Verification items for the finished model (mm, model axes). Round coordinates to 2 decimals unless told otherwise and drop trailing zeros. Write each loop counter-clockwise with the first axis right and the second up, starting at its lowest first coordinate (ties: lowest second). Pieces come first, ordered by that corner, then holes. Notation, with made-up numbers: (86, 48) - (124, 48) arc R20 cw to (124, 52) - close; hole circle Ø1 at (27.25, -11). An arc over 180 degrees is marked (long way). Answer as a JSON object with one key per item and string values.
Autodesk Fusion 360 part; units mm, degrees
sketch "Sketch15" plane through (0, 0, 0) normal (0, 1, 0) x (1, 0, 0)
  line L0 (100, 21) -> (-100, 21)
  line L1 (-100, 21) -> (-100, -21)
  line L2 (-100, -21) -> (100, -21)
  line L3 (100, -21) -> (100, 21)
  line L4 (100, 21) -> (-100, -21) construction
  line L5 (-100, 21) -> (100, -21) construction
  dimension "d41" = 200
  dimension "d42" = 42
extrude "Extrude7" add sketch "Sketch15" along normal blind 1.5
hole "Hole5" at (67.2428, 0, 13.4085) direction (0, 1, 0) diameter 3 depth 7 tip angle 118
hole "Hole6" at (75.0009, 0, 6.5047) direction (0, 1, 0) diameter 14 depth 15 tip angle 118
hole "Hole7" at (82.7411, 0, 13.4378) direction (0, 1, 0) diameter 3 depth 5 tip angle 118
hole "Hole8" at (67.2952, 0, -13.4263) direction (0, 1, 0) diameter 3 depth 6 tip angle 118
sketch "Sketch16" plane through (0, 0, 0) normal (1, 0, 0) x (0, 1, 0)
  line L0 (-56.4532, 39.0008) -> (75, 39.0008)
  line L1 (75, 39.0008) -> (75, -35)
  line L2 (75, -35) -> (-56.4532, -35)
  line L3 (-56.4532, -35) -> (-56.4532, 39.0008)
ref_plane "WorkPlane2" through (0, 9.2734, 2.0004) normal (1, 0, 0) x (0, 1, 0)
mirror "Mirror1" about plane through (0, 9.2734, 2.0004) normal (1, 0, 0) of "Hole5", "Hole7", "Hole8", "Hole6"
chamfer "Chamfer1" distance 10 angle 45 1 edges at (100, 0.75, 21)
1. Go/stop test with a flat-tipped pin: pin 1 (1.8 mm diameter, centred on x = 82.74, z = 13.44, fed in from -Y). Record where the tip stops, or that it passes through.
Completed:
{"pin 1": "passes through"}
2. Material ranges on probe 1 along X at (y, z) = (1.1, 6); probe 2 along Z at (x, y) = (66.5, 1.35); probe 3 along X at (y, z) = (1.25, 5), recorded low to high. Write a range as from..to.
Completed:
{"probe 1": "x = -100..-81.98, -68.02..68.02, 81.98..100", "probe 2": "z = -21..-14.7, -12.15..12.11, 14.71..21", "probe 3": "x = -100..-81.84, -68.16..68.16, 81.84..100"}
3. Cross-section at C-C (z = 17.5). Record the boundary of the cut face in (x, y).
Completed:
{"outline": "(-100, 0) - (93.5, 0) - (93.5, 1.5) - (-100, 1.5) - close"}
4. Cross-section at B-B (y = 0.4). Count the separate pieces of the cut face and the enclosed holes in it, plus the area to 3 significant figures.
Completed:
{"separate pieces": "1", "enclosed holes": "8", "area": "8,000 mm^2"}
5. Cross-section at A-A (z = 4). Record the boundary of the cut face in (x, y).
Completed:
{"outline": "(-100, 0) - (-81.54, 0) - (-81.54, 1.5) - (-100, 1.5) - close; (-68.46, 0) - (68.46, 0) - (68.46, 1.5) - (-68.46, 1.5) - close; (81.54, 0) - (100, 0) - (100, 1.5) - (81.54, 1.5) - close"}
6. Mould release check, pull along X, two halves, no side actions. Record for faces 1 (the face through (68.06, 0.76, 7.42)), 2 (the face through (-1, 1.5, 0)), 3 (the face through (95, 1, 16)): released by +X, released by -X, zero draft, split by the parting line, or undercut.
Completed:
{"face 1": "undercut", "face 2": "zero draft", "face 3": "released by +X"}
